Read the model definition and answer for the solid it produces. Units are mm, in the model's axes. Give positions to 0.01 mm unless a question says otherwise; leave off trailing zeros. Loops run counter-clockwise (first coordinate to the right, second up) from the corner with the lowest first, then second, coordinate; pieces in that order, holes last.
(1) Straight lines are drawn through the part: probe 1 along X at (y, z) = (-2.75, 11); probe 2 along X at (y, z) = (-4.75, 14.5); probe 3 along Y at (x, z) = (40, 18) (3 decimals). For each, find the intervals that lie inside material, in ascending order.
(2) Find section C-C, the plane y = -1.5. Write down the section's boundary in (x, z) (1 decimal), then the cut area to 3 significant figures.
(3) Find section D-D, the plane x = 40. Write down the section's boundary in (y, z) (3 decimals), then the cut area to 3 significant figures.
(4) Find section A-A, the plane x = 60. Write down the section's boundary in (y, z) (3 decimals).
(5) Find section B-B, the plane z = 2.75. Write down the section's boundary in (x, y) (3 decimals), then the cut area to 3 significant figures.
(6) Determine the mould class of faces 1 (the face through (28, -2, 0)), 2 (the face through (12.507, 0.33, 11.832)), 3 (the face through (41, -10, 12)) for opening direction Y: pulls with the +Y half, pulls with the -Y half, needs draft (parallel to the pull), parting line crosses it, or undercut.
(7) Each of these flat-tipped pins is pushed along its axis until it touches: P1, Ø1.5, axis at y = 4.5, z = 18.5, coming from the +X side; P2, Ø5, axis at x = 0, y = 0, coming from the -Z side; P3, Ø3, axis at y = -3.5, z = 17, coming from the -X side; P4, Ø3, axis at y = -3, z = 8.5, coming from the +X side. Where does it stop, or does it pass through?
```python
from build123d import *

# Parameters (mm, degrees)
SKETCH_R   = 4.25
SKETCH_R_2 = 7.5
SKETCH_R_3 = 7.575
SKETCH_R_4 = 7.625
SKETCH_R_5 = 7.75
PAD_DEPTH  = 24


with BuildPart() as part:
    # Sketch → Pad (new body)
    with BuildSketch(Plane.XY):
        with BuildLine():
            ThreePointArc((10, 0), (-7.071068, 7.071068), (0, -10))
            Line((80, -10), (0, -10))
            ThreePointArc((80, -10), (87.071068, 7.071068), (70, 0))
            ThreePointArc((70, 0), (60, 10), (50, 0))
            ThreePointArc((50, 0), (40, 10), (30, 0))
            ThreePointArc((30, 0), (20, 10), (10, 0))
        make_face()
        Circle(SKETCH_R, mode=Mode.SUBTRACT)
        with Locations((20, 0)):
            Circle(SKETCH_R_2, mode=Mode.SUBTRACT)
        with Locations((40, 0)):
            Circle(SKETCH_R_3, mode=Mode.SUBTRACT)
        with Locations((60, 0)):
            Circle(SKETCH_R_4, mode=Mode.SUBTRACT)
        with Locations((80, 0)):
            Circle(SKETCH_R_5, mode=Mode.SUBTRACT)
    extrude(amount=PAD_DEPTH)


solid = part.part
```
Entries:
1. probe 1: x = -9.61 to -3.24, 3.24 to 13.02, 26.98 to 32.94, 47.06 to 52.89, 67.11 to 72.75, 87.25 to 89.61
1. probe 2: x = -8.8 to 14.2, 25.8 to 34.1, 45.9 to 54.04, 65.96 to 73.88, 86.12 to 88.8
1. probe 3: y = -10 to -7.575, 7.575 to 10
2. outline: (-9.9, 0) - (-4, 0) - (-4, 24) - (-9.9, 24) - close; (4, 0) - (12.7, 0) - (12.7, 24) - (4, 24) - close; (27.3, 0) - (32.6, 0) - (32.6, 24) - (27.3, 24) - close; (47.4, 0) - (52.5, 0) - (52.5, 24) - (47.4, 24) - close; (67.5, 0) - (72.4, 0) - (72.4, 24) - (67.5, 24) - close; (87.6, 0) - (89.9, 0) - (89.9, 24) - (87.6, 24) - close
2. area: 771 mm2
3. outline: (-10, 0) - (-7.575, 0) - (-7.575, 24) - (-10, 24) - close; (7.575, 0) - (10, 0) - (10, 24) - (7.575, 24) - close
3. area: 116 mm2
4. outline: (-10, 0) - (-7.625, 0) - (-7.625, 24) - (-10, 24) - close; (7.625, 0) - (10, 0) - (10, 24) - (7.625, 24) - close
5. outline: (0, -10) - (80, -10) arc R10 ccw (long way) to (70, 0) arc R10 ccw to (50, 0) arc R10 ccw to (30, 0) arc R10 ccw to (10, 0) arc R10 ccw (long way) to start; hole circle Ø8.5 at (0, 0); hole circle Ø15 at (20, 0); hole circle Ø15.15 at (40, 0); hole circle Ø15.25 at (60, 0); hole circle Ø15.5 at (80, 0)
5. area: 957 mm2
6. face 1: needs draft
6. face 2: undercut
6. face 3: pulls with the -Y half
7. P1: stops at x = 89.27
7. P2: passes through
7. P3: stops at x = -9.8
7. P4: stops at x = 89.89
